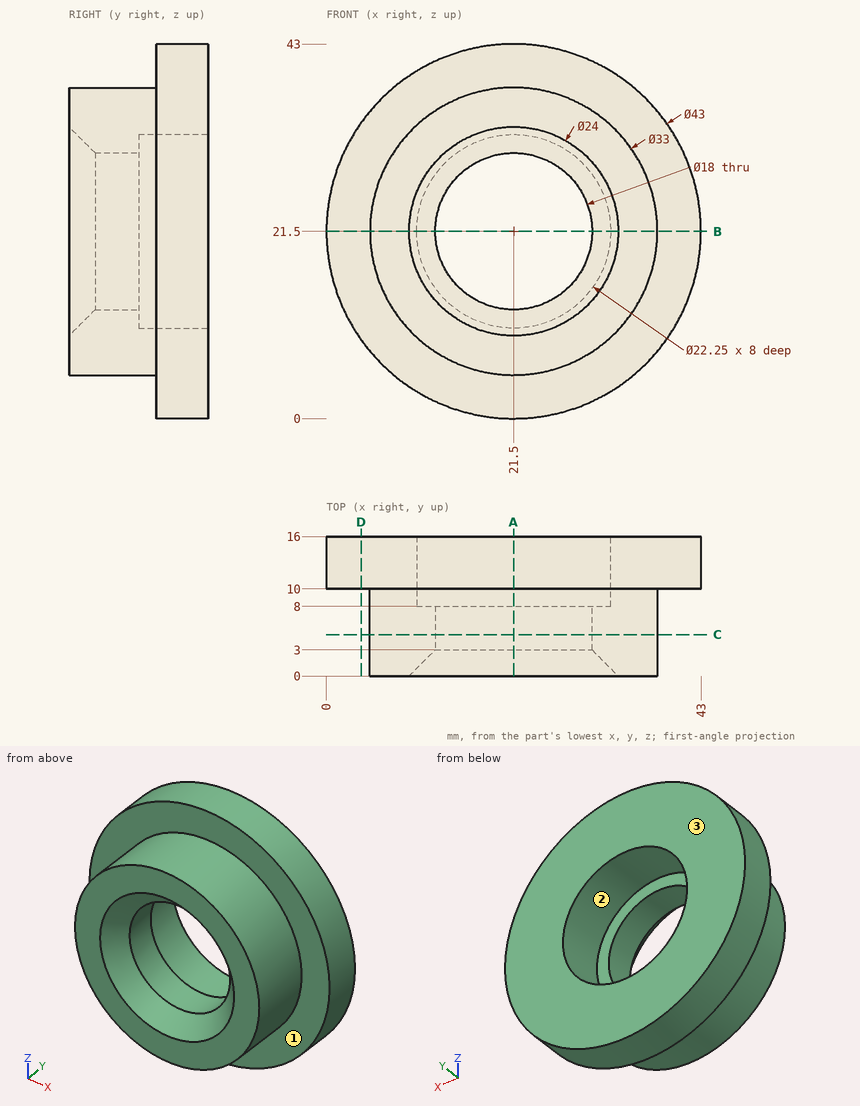
Here's the drawing with two shaded views (mm, measured from the low corner). I have some questions. A direction names the side the tool comes from. Coordinates: 2 decimals unless noted, no trailing zeros. Order: outer loops, then holes, each group sorted by start corner. A loop starts at its lowest first (then second) coordinate and runs counter-clockwise, first axis right, second up. Notation, with made-up numbers: M 42.5,-3 L 67.5,-3 A18 ccw 67.5,7 Z; hole C 72,60.5 d11. An arc over 180 degrees is marked long. Write item = value, one per line.
(1) For pin 1 Ø6.5 at (x, z) = (24.5, 18) entering from +Y; pin 2 Ø1.5 at (x, y) = (30.5, 10) entering from +Z; pin 3 Ø5 at (y, z) = (14.5, 18.5) entering from +X; pin 4 Ø8 at (x, y) = (31, 14.5) entering from +Z, each with a flat end and sliding along its axis, tell me the tip position at first contact or that it passes through.
Results are:
pin_1 = through
pin_2 = 41.35
pin_3 = 42.99
pin_4 = 42.28
(2) Suppose I cut it at B-B on z = 21.5. Please give me the cut outline in (x, y) (3 decimals), plus the area to 3 significant figures.
Results are:
outline = M 0,10 L 5,10 L 5,0 L 9.5,0 L 12.5,3 L 12.5,8 L 10.375,8 L 10.375,16 L 0,16 Z; M 30.5,3 L 33.5,0 L 38,0 L 38,10 L 43,10 L 43,16 L 32.625,16 L 32.625,8 L 30.5,8 Z
area = 257 mm2
(3) Suppose I cut it at D-D on x = 4. Please give me the cut outline in (y, z).
Results are:
outline = M 10,9.01 L 16,9.01 L 16,33.99 L 10,33.99 Z
(4) Suppose I cut it at A-A on x = 21.5. Please give me the cut outline in (y, z) (3 decimals), plus the area to 3 significant figures.
Results are:
outline = M 0,5 L 10,5 L 10,0 L 16,0 L 16,10.375 L 8,10.375 L 8,12.5 L 3,12.5 L 0,9.5 Z; M 0,33.5 L 3,30.5 L 8,30.5 L 8,32.625 L 16,32.625 L 16,43 L 10,43 L 10,38 L 0,38 Z
area = 257 mm2
(5) I need wall thicknesses on line 1 along Z through (x, y) = (21.5, 5.3); line 2 along Z through (x, y) = (21.5, 10.25) (3 decimals); line 3 along Y through (x, z) = (39.5, 16.5). Which ranges of each line are inside material? Lowest first, please. Write a range as [from, to].
Results are:
line_1 = [5, 12.5], [30.5, 38]
line_2 = [0, 10.375], [32.625, 43]
line_3 = [10, 16]
(6) For the marked faces 1, 2 and 3, which set-ups out of +Z, -Z, +X, -X, +Y, -Y let a thin tool reach every point of the face, with its end or its side?
Results are:
face_1 = -Y
face_2 = +Y
face_3 = +Z, -Z, +X, -X, +Y
(7) Suppose I cut it at C-C on y = 4.75. Please give me the cut outline in (x, z).
Results are:
outline = C 21.5,21.5 d33; hole C 21.5,21.5 d18
